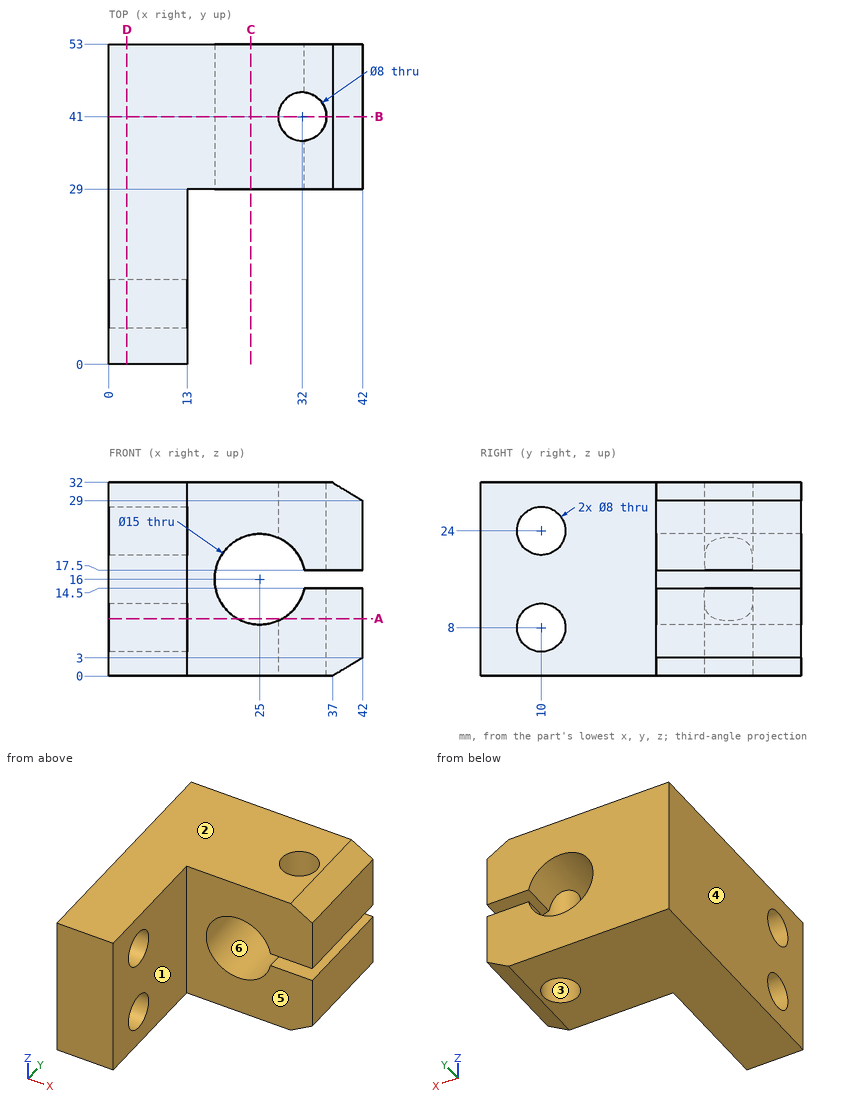
Study the drawing (mm; zero at the part's minimum x, y, z) and answer. A direction names the side the tool comes from. Round coordinates to 2 decimals unless told otherwise and drop trailing zeros. Write each loop counter-clockwise with the first axis right and the second up, starting at its lowest first coordinate (ties: lowest second). Pieces come first, ordered by that corner, then holes. Notation, with made-up numbers: (50.5, 1.25) -> (101.5, 1.25) arc R6 ccw to (101.5, 11.25) -> close; hole circle Ø2 at (-18.75, 35.5). An arc over 180 degrees is marked (long way). Use CSV: the item, a comma, the result in double quotes. Start each with the question number.
(1) Section A-A on z = 9.5 is taken. Give the vertices of the cut face in (x, y), then the cut area to 3 significant figures.
(2) Each of these flat-tipped pins is pushed along its axis until it touches: pin 1 (2 mm diameter, centred on x = 32, z = 14, fed in from -Y); pin 2 (12 mm diameter, centred on y = 20.5, z = 15.5, fed in from +X). Where does it stop, or does it pass through?
(3) Section C-C on x = 23.5 is taken. Give the vertices of the cut face in (y, z).
(4) Section D-D on x = 3 is taken. Give the vertices of the cut face in (y, z), then the cut area to 3 significant figures.
(5) Which of the six approach directions +Z, -Z, +X, -X, +Y, -Y give full straight-line access (tool end or side, diameter ignored) to the marked faces 5 and 6?
(6) Section B-B on y = 41 is taken. Give the vertices of the cut face in (x, z).
(7) Consider L1, parallel to Y at x = 32, z = 25; L2, parallel to Z at x = 25, y = 47; L3, parallel to Y at x = 10, z = 24. Determine where each line is inside the solid, lowest interval first. Write a range as from..to.
(8) The mould has two halves that part along X. Classify the marked faces 1, 2, 3 and 4: released by +X, released by -X, zero draft, split by the parting line, or undercut.
A:
1,outline,"(0, 0) -> (13, 0) -> (13, 6.29) -> (0, 6.29) -> close; (0, 13.71) -> (13, 13.71) -> (13, 29) -> (21.26, 29) -> (21.26, 53) -> (0, 53) -> close; (28.74, 29) -> (42, 29) -> (42, 53) -> (28.74, 53) -> (28.74, 43.32) arc R4 cw (long way) to (28.74, 38.68) -> close"
1,area,"1,060 mm²"
2,pin 1,"stops at y = 29"
2,pin 2,"stops at x = 13"
3,outline,"(29, 0) -> (53, 0) -> (53, 8.65) -> (29, 8.65) -> close; (29, 23.35) -> (53, 23.35) -> (53, 32) -> (29, 32) -> close"
4,outline,"(0, 0) -> (53, 0) -> (53, 32) -> (0, 32) -> close; hole circle Ø8 at (10, 8); hole circle Ø8 at (10, 24)"
4,area,"1,600 mm²"
5,face 5,"+Z, -Z, +X, -Y"
5,face 6,"+Y, -Y"
6,outline,"(0, 0) -> (28, 0) -> (28, 9.13) arc R7.5 cw (long way) to (28, 22.87) -> (28, 32) -> (0, 32) -> close; (36, 0) -> (37, 0) -> (42, 3) -> (42, 14.5) -> (36, 14.5) -> close; (36, 17.5) -> (42, 17.5) -> (42, 29) -> (37, 32) -> (36, 32) -> close"
7,L1,"y = 29..37, 45..53"
7,L2,"z = 0..8.5, 23.5..32"
7,L3,"y = 0..6, 14..53"
8,face 1,"released by +X"
8,face 2,"zero draft"
8,face 3,"undercut"
8,face 4,"released by -X"
